from build123d import *

# Parameters (mm, degrees)
SKETCH1_R           = 2.1
BOSS_EXTRUDE1_DEPTH = 500
SKETCH2_W           = 72.199541976
SKETCH2_H           = 58.054703084
CUT_EXTRUDE2_DEPTH  = 189.7888


with BuildPart() as part:
    # Sketch1 → Boss-Extrude1 (new body)
    with BuildSketch(Plane.XY):
        with BuildLine():
            Line((4.58, -20), (9.5, -20))
            ThreePointArc((9.5, -20), (9.853553391, -19.853553391), (10, -19.5))
            Line((10, -19.5), (10, -14.58))
            Line((10, -14.58), (8.545, -13.125))
            Line((8.545, -13.125), (8.2, -13.125))
            Line((8.2, -13.125), (8.2, -15.5))
            Line((8.2, -15.5), (6.560660172, -15.5))
            Line((6.560660172, -15.5), (3.9, -12.839339828))
            Line((3.9, -12.839339828), (3.9, -10.21))
            Line((3.9, -10.21), (3.69, -10))
            Line((3.69, -10), (3.9, -9.79))
            Line((3.9, -9.79), (3.9, -7.160660172))
            Line((3.9, -7.160660172), (6.560660172, -4.5))
            Line((6.560660172, -4.5), (8.2, -4.5))
            Line((8.2, -4.5), (8.2, -6.875))
            Line((8.2, -6.875), (8.545, -6.875))
            Line((8.545, -6.875), (10, -5.42))
            Line((10, -5.42), (10, 5.42))
            Line((10, 5.42), (8.545, 6.875))
            Line((8.545, 6.875), (8.2, 6.875))
            Line((8.2, 6.875), (8.2, 4.5))
            Line((8.2, 4.5), (6.560660172, 4.5))
            Line((6.560660172, 4.5), (3.9, 7.160660172))
            Line((3.9, 7.160660172), (3.9, 9.79))
            Line((3.9, 9.79), (3.69, 10))
            Line((3.69, 10), (3.9, 10.21))
            Line((3.9, 10.21), (3.9, 12.839339828))
            Line((3.9, 12.839339828), (6.560660172, 15.5))
            Line((6.560660172, 15.5), (8.2, 15.5))
            Line((8.2, 15.5), (8.2, 13.125))
            Line((8.2, 13.125), (8.545, 13.125))
            Line((8.545, 13.125), (10, 14.58))
            Line((10, 14.58), (10, 19.5))
            ThreePointArc((10, 19.5), (9.853553391, 19.853553391), (9.5, 20))
            Line((9.5, 20), (4.58, 20))
            Line((4.58, 20), (3.125, 18.545))
            Line((3.125, 18.545), (3.125, 18.2))
            Line((3.125, 18.2), (5.5, 18.2))
            Line((5.5, 18.2), (5.5, 16.560660172))
            Line((5.5, 16.560660172), (2.839339828, 13.9))
            Line((2.839339828, 13.9), (0.21, 13.9))
            Line((0.21, 13.9), (0, 13.69))
            Line((0, 13.69), (-0.21, 13.9))
            Line((-0.21, 13.9), (-2.839339828, 13.9))
            Line((-2.839339828, 13.9), (-5.5, 16.560660172))
            Line((-5.5, 16.560660172), (-5.5, 18.2))
            Line((-5.5, 18.2), (-3.125, 18.2))
            Line((-3.125, 18.2), (-3.125, 18.545))
            Line((-3.125, 18.545), (-4.58, 20))
            Line((-4.58, 20), (-9.5, 20))
            ThreePointArc((-9.5, 20), (-9.853553391, 19.853553391), (-10, 19.5))
            Line((-10, 19.5), (-10, 14.58))
            Line((-10, 14.58), (-8.545, 13.125))
            Line((-8.545, 13.125), (-8.2, 13.125))
            Line((-8.2, 13.125), (-8.2, 15.5))
            Line((-8.2, 15.5), (-6.560660172, 15.5))
            Line((-6.560660172, 15.5), (-3.9, 12.839339828))
            Line((-3.9, 12.839339828), (-3.9, 10.21))
            Line((-3.9, 10.21), (-3.69, 10))
            Line((-3.69, 10), (-3.9, 9.79))
            Line((-3.9, 9.79), (-3.9, 7.160660172))
            Line((-3.9, 7.160660172), (-6.560660172, 4.5))
            Line((-6.560660172, 4.5), (-8.2, 4.5))
            Line((-8.2, 4.5), (-8.2, 6.875))
            Line((-8.2, 6.875), (-8.545, 6.875))
            Line((-8.545, 6.875), (-10, 5.42))
            Line((-10, 5.42), (-10, -5.42))
            Line((-10, -5.42), (-8.545, -6.875))
            Line((-8.545, -6.875), (-8.2, -6.875))
            Line((-8.2, -6.875), (-8.2, -4.5))
            Line((-8.2, -4.5), (-6.560660172, -4.5))
            Line((-6.560660172, -4.5), (-3.9, -7.160660172))
            Line((-3.9, -7.160660172), (-3.9, -9.79))
            Line((-3.9, -9.79), (-3.69, -10))
            Line((-3.69, -10), (-3.9, -10.21))
            Line((-3.9, -10.21), (-3.9, -12.839339828))
            Line((-3.9, -12.839339828), (-6.560660172, -15.5))
            Line((-6.560660172, -15.5), (-8.2, -15.5))
            Line((-8.2, -15.5), (-8.2, -13.125))
            Line((-8.2, -13.125), (-8.545, -13.125))
            Line((-8.545, -13.125), (-10, -14.58))
            Line((-10, -14.58), (-10, -19.5))
            ThreePointArc((-10, -19.5), (-9.853553391, -19.853553391), (-9.5, -20))
            Line((-9.5, -20), (-4.58, -20))
            Line((-4.58, -20), (-3.125, -18.545))
            Line((-3.125, -18.545), (-3.125, -18.2))
            Line((-3.125, -18.2), (-5.5, -18.2))
            Line((-5.5, -18.2), (-5.5, -16.560660172))
            Line((-5.5, -16.560660172), (-2.839339828, -13.9))
            Line((-2.839339828, -13.9), (-0.21, -13.9))
            Line((-0.21, -13.9), (0, -13.69))
            Line((0, -13.69), (0.21, -13.9))
            Line((0.21, -13.9), (2.839339828, -13.9))
            Line((2.839339828, -13.9), (5.5, -16.560660172))
            Line((5.5, -16.560660172), (5.5, -18.2))
            Line((5.5, -18.2), (3.125, -18.2))
            Line((3.125, -18.2), (3.125, -18.545))
            Line((3.125, -18.545), (4.58, -20))
        make_face()
        with Locations((0, -10)):
            Circle(SKETCH1_R, mode=Mode.SUBTRACT)
        Polygon((-6.239339828, -2.7), (-8.2, -2.7), (-8.2, 2.7), (-6.239339828, 2.7), (-2.839339828, 6.1), (2.839339828, 6.1), (6.239339828, 2.7), (8.2, 2.7), (8.2, -2.7), (6.239339828, -2.7), (2.839339828, -6.1), (-2.839339828, -6.1), align=None, mode=Mode.SUBTRACT)
        with Locations((0, 10)):
            Circle(SKETCH1_R, mode=Mode.SUBTRACT)
    extrude(amount=BOSS_EXTRUDE1_DEPTH)

    # Sketch2 → Cut-Extrude2 (cut)
    with BuildSketch(Plane(origin=(0, 0, 0), x_dir=(-1, 0, 0), z_dir=(0, 0, -1))):
        with Locations((-4.42817029, -8.078427536)):
            Rectangle(SKETCH2_W, SKETCH2_H)
    extrude(amount=-CUT_EXTRUDE2_DEPTH, mode=Mode.SUBTRACT)


solid = part.part
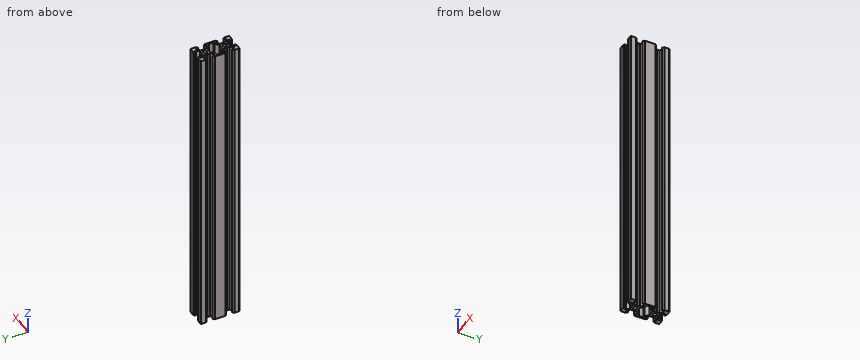
Check sheet for the modelled part. Datum: model origin and axes. Units: mm. Round coordinates to 2 decimals unless told otherwise and drop trailing zeros.
(1) Cross-section at A-A, the plane z = 245. State how many separate pieces and enclosed holes the cut face has, and give its area (3 significant figures).
(2) Scan lines: probe 1 along Y at (x, z) = (0, 274); probe 2 along Y at (x, z) = (-0.5, 380); probe 3 along X at (y, z) = (15, 470). Record each from-to range of solid material in increasing order.
(3) Go/stop test with flat-tipped pins: P1, Ø1.3, axis at y = 9, z = 283, coming from the -X side; P2, Ø8, axis at x = 0.5, z = 317.5, coming from the +Y side; P3, Ø1.7, axis at x = 0, z = 366, coming from the -Y side. Record where each tip stops, or that it passes through.
Check sheet entries:
1. separate pieces: 1
1. enclosed holes: 3
1. area: 300 mm2
2. probe 1: y = -13.69 to -12.1, -7.9 to -6.1, 6.1 to 7.9, 12.1 to 13.69
2. probe 2: y = -13.9 to -12.04, -7.96 to -6.1, 6.1 to 7.96, 12.04 to 13.9
2. probe 3: x = -10 to -8.2, -6.06 to -3.94, 3.94 to 6.06, 8.2 to 10
3. P1: stops at x = -3.9
3. P2: stops at y = 19.92
3. P3: stops at y = -13.9
